Autodesk Inventor part; units mm, degrees
ref_plane "YZ Plane" through (0, 0, 0) normal (1, 0, 0) x (0, 1, 0)
ref_plane "XZ Plane" through (0, 0, 0) normal (0, 1, 0) x (-1, 0, 0)
ref_plane "XY Plane" through (0, 0, 0) normal (0, 0, 1) x (1, 0, 0)
sketch "Sketch1" plane through (0, 0, 0) normal (0, 1, 0) x (-1, 0, 0)
  line L0 (0, 0) -> (170, 0)
  line L1 (170, 0) -> (170, -140)
  line L2 (170, -140) -> (0, -140)
  line L3 (0, -140) -> (0, 0)
  line L4 (165.2375, -4.7625) -> (4.7625, -4.7625)
  line L5 (4.7625, -4.7625) -> (4.7625, -135.2375)
  line L6 (4.7625, -135.2375) -> (165.2375, -135.2375)
  line L7 (165.2375, -135.2375) -> (165.2375, -4.7625)
  dimension "d0" = 170
  dimension "d1" = 140
  dimension "d2" = 4.7625
  dimension "d3" = 4.7625
  dimension "d4" = 4.7625
  dimension "d5" = 4.7625
  dimension "d6" = 4.7625
extrude "Extrusion1" add sketch "Sketch1" along normal blind 30
sketch "Sketch2" plane through (0, 30, 0) normal (0, 1, 0) x (1, 0, 0)
  line L0 (-4.7625, 4.7625) -> (-165.2375, 4.7625)
  line L1 (-165.2375, 4.7625) -> (-4.7625, 4.7625)
  line L2 (-4.7625, 4.7625) -> (-4.7625, 135.2375)
  line L3 (-4.7625, 135.2375) -> (-165.2375, 135.2375)
  line L4 (-165.2375, 135.2375) -> (-165.2375, 4.7625)
  point P0 (0, 0)
extrude "Extrusion2" add sketch "Sketch2" against normal blind 12.7
sketch "Sketch3" plane through (0, 30, 0) normal (0, 1, 0) x (1, 0, 0)
  line L0 (-165.2375, 135.2375) -> (-165.2375, 4.7625)
  line L1 (-4.7625, 4.7625) -> (-4.7625, 135.2375)
  line L2 (-165.2375, 4.7625) -> (-4.7625, 4.7625)
  line L3 (-4.7625, 4.7625) -> (-4.7625, 135.2375)
  line L4 (-4.7625, 135.2375) -> (-165.2375, 135.2375)
  line L5 (-165.2375, 135.2375) -> (-165.2375, 4.7625)
  point P0 (0, 0)
extrude "Extrusion3" add sketch "Sketch3" along normal blind 0.0254
properties part number "OpticalDeviceLookThroughPart" material "Glass"
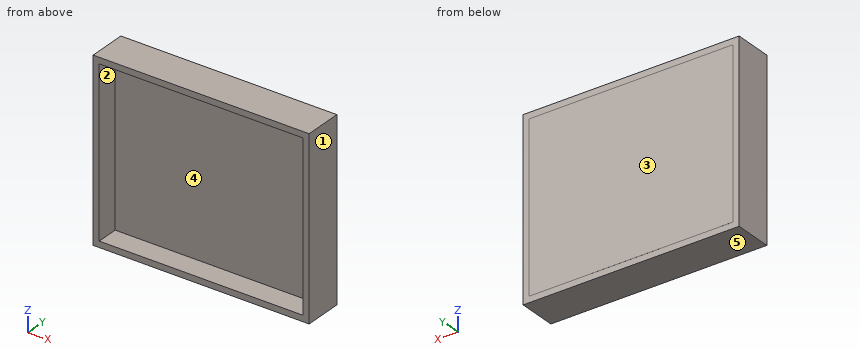
Geometry check sheet. Reference: the model listing, model coordinates, mm. Face numbers are marked on the shaded views. A direction names the side the tool comes from. Round coordinates to 2 decimals unless told otherwise and drop trailing zeros. Order: outer loops, then holes, each group sorted by start corner. A loop starts at its lowest first (then second) coordinate and runs counter-clockwise, first axis right, second up. Notation, with made-up numbers: (47.5, 42.25) -> (104.5, 42.25) arc R12 ccw to (104.5, 58.25) -> close; hole circle Ø7 at (-32.75, 40.5). An arc over 180 degrees is marked (long way). Use one line per item in the form item = value.
1. Set-up check for the marked faces 4 and 5: record each of +Z, -Z, +X, -X, +Y, -Y from which the full face is reachable in a straight line by a thin tool's end or side.
Working result:
face_4 = -Y
face_5 = -Z, +X, -X, +Y, -Y
2. Mould release check, pull along X, two halves, no side actions. Record for the marked faces 1, 2 and 3: pulls with the +X half, pulls with the -X half, needs draft (parallel to the pull), parting line crosses it, or undercut.
Working result:
face_1 = pulls with the +X half
face_2 = undercut
face_3 = needs draft
3. Scan lines: line 1 along X through (y, z) = (11.5, -16); line 2 along Z through (x, y) = (-29.5, 4); line 3 along Y through (x, z) = (-139, -114). Record each from-to range of solid material in increasing order. Write a range as from..to.
Working result:
line_1 = -170..-165.24, -4.76..0
line_2 = -140..-135.24, -4.76..0
line_3 = 17.3..30.03
4. Go/stop test with a flat-tipped pin: pin 1 (8 mm diameter, centred on x = -75, z = -105.5, fed in from -Y). Record where the tip stops, or that it passes through.
Working result:
pin_1 = 17.3
5. Cross-section at B-B, the plane y = 15. Enter the section's corners in (x, z).
Working result:
outline = (-170, -140) -> (0, -140) -> (0, 0) -> (-170, 0) -> close; hole (-165.24, -135.24) -> (-4.76, -135.24) -> (-4.76, -4.76) -> (-165.24, -4.76) -> close
